Autodesk Inventor part; units mm, degrees
ref_plane "YZ Plane" through (0, 0, 0) normal (1, 0, 0) x (0, 1, 0)
ref_plane "XZ Plane" through (0, 0, 0) normal (0, 1, 0) x (-1, 0, 0)
ref_plane "XY Plane" through (0, 0, 0) normal (0, 0, 1) x (1, 0, 0)
ref_plane "Work Plane1" through (1.3068, 17.1014, 0) normal (0, 0, 1) x (1, 0, 0)
sketch "Sketch2" plane through (1.3068, 17.1014, 0) normal (0, 0, 1) x (1, 0, 0)
  line L0 (-22, -19.25) -> (-22, 19.25)
  line L1 (-22, 19.25) -> (22, 19.25)
  line L2 (22, -19.25) -> (-22, -19.25)
  line L3 (-22, 19.25) -> (22, 19.25)
  line L4 (22, 19.25) -> (22, -19.25)
  line L5 (-22, 19.25) -> (22, 19.25)
  line L6 (-22, 19.25) -> (-18.19, 19.25)
  line L7 (-22, 15.44) -> (-22, 19.25)
  line L8 (-22, -19.25) -> (-18.19, -19.25)
  line L9 (22, -19.25) -> (18.19, -19.25)
  line L10 (22, -15.44) -> (22, -19.25)
  line L11 (22, 15.44) -> (22, 19.25)
  line L12 (22, 19.25) -> (18.19, 19.25)
  line L13 (18.19, 17.345) -> (-18.19, 17.345)
  line L14 (-18.19, 17.345) -> (-18.19, 15.44)
  line L15 (-18.19, 15.44) -> (18.19, 15.44)
  line L16 (18.19, 15.44) -> (18.19, 17.345)
  line L17 (18.19, -17.345) -> (-18.19, -17.345)
  line L18 (-18.19, -17.345) -> (-18.19, -15.44)
  line L19 (-18.19, -15.44) -> (18.19, -15.44)
  line L20 (18.19, -15.44) -> (18.19, -17.345)
  circle A0 centre (-24.1175, -24.3391) radius 2.25
  circle A1 centre (-24.2491, 24.2487) radius 2.25
  circle A2 centre (24.2419, 24.2487) radius 2.25
  circle A3 centre (24.2419, -24.2423) radius 2.25
  line L21 (15.2616, -22.247) -> (15.2616, -26.057)
  arc A4 (15.2616, -26.057) -> (18.4366, -29.232) centre (18.4366, -26.057) ccw
  line L22 (18.4366, -29.232) -> (26.0566, -29.232)
  arc A5 (26.0566, -29.232) -> (29.2316, -26.057) centre (26.0566, -26.057) ccw
  line L23 (29.2316, -26.057) -> (29.2316, -15.262)
  line L24 (29.2316, -15.262) -> (18.3723, -15.262)
  line L25 (18.3723, 15.2684) -> (26.0566, 15.2684)
  arc A6 (26.0566, 15.2684) -> (29.2316, 18.4434) centre (26.0566, 18.4434) ccw
  line L26 (29.2316, 18.4434) -> (29.2316, 26.0634)
  arc A7 (29.2316, 26.0634) -> (26.0566, 29.2384) centre (26.0566, 26.0634) ccw
  line L27 (26.0566, 29.2384) -> (18.4366, 29.2384)
  line L28 (15.2616, 26.0634) -> (15.2616, 22.2534)
  arc A8 (18.4366, 29.2384) -> (15.2616, 26.0634) centre (18.4366, 26.0634) ccw
  line L29 (-26.0638, 15.2684) -> (-15.2688, 15.2684)
  arc A9 (-29.2388, 18.4434) -> (-26.0638, 15.2684) centre (-26.0638, 18.4434) ccw
  line L30 (-29.2388, 26.0634) -> (-29.2388, 18.4434)
  arc A10 (-26.0638, 29.2384) -> (-29.2388, 26.0634) centre (-26.0638, 26.0634) ccw
  line L31 (-18.4438, 29.2384) -> (-26.0638, 29.2384)
  arc A11 (-15.2688, 26.0634) -> (-18.4438, 29.2384) centre (-18.4438, 26.0634) ccw
  line L32 (-15.2688, 22.2534) -> (-15.2688, 26.0634)
  line L33 (-15.2688, -26.057) -> (-15.2688, -22.247)
  arc A12 (-18.4438, -29.232) -> (-15.2688, -26.057) centre (-18.4438, -26.057) ccw
  line L34 (-26.0638, -29.232) -> (-18.4438, -29.232)
  arc A13 (-29.2388, -26.057) -> (-26.0638, -29.232) centre (-26.0638, -26.057) ccw
  line L35 (-29.2388, -18.437) -> (-29.2388, -26.057)
  arc A14 (-26.0638, -15.262) -> (-29.2388, -18.437) centre (-26.0638, -18.437) ccw
  line L36 (-15.2688, -15.262) -> (-26.0638, -15.262)
  line L37 (-15.2688, -22.247) -> (-15.2688, -19.25)
  line L38 (15.2616, -22.247) -> (15.2616, -19.25)
  line L39 (15.2616, 22.2534) -> (15.2616, 19.25)
  line L40 (-15.2688, 22.2534) -> (-15.2688, 19.25)
  point P0 (-1.3068, -17.1014)
  point P1 (0, 0)
  point P2 (22, -15.262)
  point P3 (18.19, -19.25)
  point P4 (15.2616, 19.25)
  point P5 (22, 15.2684)
  point P6 (-22, 15.2684)
  point P7 (-22, -15.262)
extrude "Extrusion2" add sketch "Sketch2" along normal blind 2.54
sketch "Sketch4" plane through (1.3068, 17.1014, 0) normal (0, 0, -1) x (-1, 0, 0)
  line L0 (22, 21.155) -> (22, 19.25)
  arc A0 (22, 21.155) -> (18.19, 21.155) centre (20.095, 21.155) ccw
  line L1 (18.19, 19.25) -> (18.19, 21.155)
  line L2 (22, 19.25) -> (23.905, 19.25)
  arc A1 (23.905, 15.44) -> (23.905, 19.25) centre (23.905, 17.345) ccw
  line L3 (23.905, 15.44) -> (22, 15.44)
  line L4 (-23.905, 19.25) -> (-22, 19.25)
  arc A2 (-23.905, 19.25) -> (-23.905, 15.44) centre (-23.905, 17.345) ccw
  line L5 (-22, 15.44) -> (-23.905, 15.44)
  line L6 (-22, 19.25) -> (-22, 21.155)
  arc A3 (-18.19, 21.155) -> (-22, 21.155) centre (-20.095, 21.155) ccw
  line L7 (-18.19, 21.155) -> (-18.19, 19.25)
  line L8 (-23.905, -15.44) -> (-22, -15.44)
  arc A4 (-23.905, -15.44) -> (-23.905, -19.25) centre (-23.905, -17.345) ccw
  line L9 (-22, -19.25) -> (-23.905, -19.25)
  line L10 (-22, -21.155) -> (-22, -19.25)
  arc A5 (-22, -21.155) -> (-18.19, -21.155) centre (-20.095, -21.155) ccw
  line L11 (-18.19, -19.25) -> (-18.19, -21.155)
  line L12 (18.19, -21.155) -> (18.19, -19.25)
  arc A6 (18.19, -21.155) -> (22, -21.155) centre (20.095, -21.155) ccw
  line L13 (22, -19.25) -> (22, -21.155)
  line L14 (23.905, -19.25) -> (22, -19.25)
  line L15 (22, -15.44) -> (23.905, -15.44)
  arc A7 (23.905, -19.25) -> (23.905, -15.44) centre (23.905, -17.345) ccw
  line L16 (22, -15.44) -> (22, -19.25)
  line L17 (18.19, -19.25) -> (22, -19.25)
  line L18 (-22, -19.25) -> (-18.19, -19.25)
  line L19 (-22, -15.44) -> (-22, -19.25)
  line L20 (-22, 19.25) -> (-22, 15.44)
  line L21 (-22, 19.25) -> (-18.19, 19.25)
  line L22 (18.19, 19.25) -> (22, 19.25)
  line L23 (22, 21.155) -> (22, 19.25)
  line L24 (22, 15.44) -> (22, 19.25)
  point P0 (1.3068, -17.1014)
extrude "Extrusion3" add sketch "Sketch4" along normal blind 11.545
properties part number "cover" material "ABS Plastic"
Source: CAD feature listing. Evaluate the final solid. Frame: model axes, mm. A direction names the side the tool comes from. Round coordinates to 2 decimals unless told otherwise and drop trailing zeros. Write each loop counter-clockwise with the first axis right and the second up, starting at its lowest first coordinate (ties: lowest second). Pieces come first, ordered by that corner, then holes. Notation, with made-up numbers: (-18.75, -5) - (-7.75, -5) arc R21 cw to (-7.75, 16) - close; hole circle Ø10 at (65, 79.5). An arc over 180 degrees is marked (long way). Use CSV: the item, a comma, the result in double quotes. Start each with the question number.
(1) Cut plane B-B, the plane y = 37.5. Return loops of the section in (x, z) (3 decimals), and give its area (3 significant figures).
(2) Material intervals for probe 1 along X at (y, z) = (41.5, 1.5); probe 2 along X at (y, z) = (-3, -0.25); probe 3 along Y at (x, z) = (25, -0.25), sorted ascending. Write a range as [from, to].
(3) Mould query, pull axis X, two halves, no side actions, for faces 4 (the face through (-27.027, 45.385, 1.252)), 5 (the face through (16.568, 40, 1)), 6 (the face through (-22, 1.661, -6)). Classes: pulls with the +X half, pulls with the -X half, needs draft (parallel to the pull), parting line crosses it, or undercut.
(4) Set-up query: faces 1 (the face through (23.307, 34, -6)), 2 (the face through (-16.883, -3, -6)), 3 (the face through (1, 36.351, 1)). Return all of +Z, -Z, +X, -X, +Y, -Y with unobstructed straight access to the full face (end or side cutting, diameter ignored); none if empty.
(5) Cut plane D-D, the plane y = 26. Return loops of the section in (x, z), and give its area (3 significant figures).
(6) Cut plane C-C, the plane x = 1.5. Return loops of the section in (y, z), and give its area (3 significant figures).
(7) First-contact query: pin 1 Ø5 at (x, y) = (17.5, 18) entering from -Z; pin 2 Ø1.3 at (x, z) = (-5, 1) entering from -Y; pin 3 Ø1.3 at (x, z) = (6.5, 1) entering from +Y. Flat tips, straight axial feed; report the tip coordinate or a pass-through.
Geometry says:
1,outline,"(-27.932, 0) - (-20.693, 0) - (-20.693, -11.545) - (-16.883, -11.545) - (-16.883, 0) - (-13.962, 0) - (-13.962, 2.54) - (-27.932, 2.54) - close; (16.568, 0) - (19.497, 0) - (19.497, -11.545) - (23.307, -11.545) - (23.307, 0) - (30.538, 0) - (30.538, 2.54) - (16.568, 2.54) - close"
1,area,"159 mm²"
2,probe 1,"[-27.93, -25.19], [-20.7, -13.96], [16.57, 23.3], [27.79, 30.54]"
2,probe 2,"[-20.69, -16.88], [19.5, 23.31]"
2,probe 3,"[-2.15, 1.66], [32.54, 36.35]"
3,face 4,"pulls with the -X half"
3,face 5,"undercut"
3,face 6,"needs draft"
4,face 1,"-Z"
4,face 2,"-Z, +Y, -Y"
4,face 3,"+Z, -Z, +Y"
5,outline,"(-20.69, 0) - (23.31, 0) - (23.31, 2.54) - (-20.69, 2.54) - close"
5,area,"112 mm²"
6,outline,"(-2.15, 0) - (-0.24, 0) - (-0.24, 2.54) - (-2.15, 2.54) - close; (1.66, 0) - (32.54, 0) - (32.54, 2.54) - (1.66, 2.54) - close; (34.45, 0) - (36.35, 0) - (36.35, 2.54) - (34.45, 2.54) - close"
6,area,"88.1 mm²"
7,pin 1,"z = 0"
7,pin 2,"y = -2.15"
7,pin 3,"y = 36.35"
